from build123d import *

# Parameters (mm, degrees)
F0_R     = 38.89375
F0_R_2   = 6.35
F1_DEPTH = 4.7625
F2_R     = 38.89375
F2_R_2   = 28.575
F3_DEPTH = 1.5875
F4_R     = 6.35
F5_DEPTH = 15.875
F7_DEPTH = 12.7
F7_TAPER = 5
F8_R     = 3.175
F9_DEPTH = 12.7


with BuildPart() as f1:
    # F0 (on Front) → F1 (new body)
    with BuildSketch(Plane.XZ):
        Circle(F0_R)
        Circle(F0_R_2, mode=Mode.SUBTRACT)
    extrude(amount=F1_DEPTH)

    # F2 (on face) → F3 (join)
    with BuildSketch(Plane.XZ.offset(4.7625)):
        Circle(F2_R)
        Circle(F2_R_2, mode=Mode.SUBTRACT)
    extrude(amount=F3_DEPTH)

    # F4 (on face) → F5 (join)
    with BuildSketch(Plane(origin=(0, 0, 0), x_dir=(-1, 0, 0), z_dir=(0, 1, 0))):
        with BuildLine():
            Line((-15.875, -79.375), (15.875, -79.375))
            Line((15.875, -79.375), (15.875, -35.5064524286))
            ThreePointArc((15.875, -35.5064524286), (0, -38.89375), (-15.875, -35.5064524286))
            Line((-15.875, -35.5064524286), (-15.875, -79.375))
        make_face()
        with BuildLine():
            ThreePointArc((-15.875, -35.5064524286), (0, -38.89375), (15.875, -35.5064524286))
            Line((15.875, -35.5064524286), (15.875, 0))
            ThreePointArc((15.875, 0), (4.9e-09, -15.875), (-15.875, -9.8e-09))
            Line((-15.875, -9.8e-09), (-15.875, -35.5064524286))
        make_face()
        with BuildLine():
            ThreePointArc((-15.875, -9.8e-09), (4.9e-09, -15.875), (15.875, 0))
            ThreePointArc((15.875, 0), (-4.9e-09, 15.875), (-15.875, -9.8e-09))
        make_face()
        Circle(F4_R, mode=Mode.SUBTRACT)
    extrude(amount=F5_DEPTH)

    # F6 (on face) → F7 (cut)
    with BuildSketch(Plane(origin=(0, 15.875, 0), x_dir=(-1, 0, 0), z_dir=(0, 1, 0))):
        with BuildLine():
            ThreePointArc((-6.35, -60.325), (-4.4901280605, -64.8151280605), (0, -66.675))
            Line((0, -66.675), (0, -60.325))
            Line((0, -60.325), (-6.35, -60.325))
        make_face()
        with BuildLine():
            Line((0, -60.325), (0, -66.675))
            ThreePointArc((0, -66.675), (4.4901280605, -64.8151280605), (6.35, -60.325))
            Line((6.35, -60.325), (0, -60.325))
        make_face()
        with BuildLine():
            Line((-6.35, -60.325), (0, -60.325))
            Line((0, -60.325), (0, -53.975))
            ThreePointArc((0, -53.975), (-4.4901280605, -55.8348719395), (-6.35, -60.325))
        make_face()
        with BuildLine():
            Line((0, -53.975), (0, -60.325))
            Line((0, -60.325), (6.35, -60.325))
            ThreePointArc((6.35, -60.325), (4.4901280605, -55.8348719395), (0, -53.975))
        make_face()
        with BuildLine():
            Line((-6.35, -22.225), (-6.35, -60.325))
            ThreePointArc((-6.35, -60.325), (-4.4901280605, -55.8348719395), (0, -53.975))
            Line((0, -53.975), (0, -28.575))
            ThreePointArc((0, -28.575), (-4.4901280605, -26.7151280605), (-6.35, -22.225))
        make_face()
        with BuildLine():
            ThreePointArc((0, -53.975), (4.4901280605, -55.8348719395), (6.35, -60.325))
            Line((6.35, -60.325), (6.35, -22.225))
            ThreePointArc((6.35, -22.225), (4.4901280605, -26.7151280605), (0, -28.575))
            Line((0, -28.575), (0, -53.975))
        make_face()
        with BuildLine():
            ThreePointArc((0, -15.875), (-4.4901280605, -17.7348719395), (-6.35, -22.225))
            Line((-6.35, -22.225), (0, -22.225))
            Line((0, -22.225), (0, -15.875))
        make_face()
        with BuildLine():
            Line((0, -22.225), (-6.35, -22.225))
            ThreePointArc((-6.35, -22.225), (-4.4901280605, -26.7151280605), (0, -28.575))
            Line((0, -28.575), (0, -22.225))
        make_face()
        with BuildLine():
            ThreePointArc((0, -28.575), (4.4901280605, -26.7151280605), (6.35, -22.225))
            Line((6.35, -22.225), (0, -22.225))
            Line((0, -22.225), (0, -28.575))
        make_face()
        with BuildLine():
            Line((0, -22.225), (6.35, -22.225))
            ThreePointArc((6.35, -22.225), (4.4901280605, -17.7348719395), (0, -15.875))
            Line((0, -15.875), (0, -22.225))
        make_face()
    extrude(amount=-F7_DEPTH, taper=F7_TAPER, mode=Mode.SUBTRACT)

    # F8 (on face) → F9 (cut)
    with BuildSketch(Plane(origin=(0, 15.875, 0), x_dir=(-1, 0, 0), z_dir=(0, 1, 0))):
        with BuildLine():
            ThreePointArc((3.175, -11.1125), (2.2450640303, -8.8674359697), (0, -7.9375))
            Line((0, -7.9375), (0, -14.2875))
            ThreePointArc((0, -14.2875), (2.2450640303, -13.3575640303), (3.175, -11.1125))
        make_face()
        with BuildLine():
            ThreePointArc((12.7, -69.85), (9.525, -66.675), (6.35, -69.85))
            ThreePointArc((6.35, -69.85), (9.525, -73.025), (12.7, -69.85))
        make_face()
        with Locations((-9.525, -69.85)):
            Circle(F8_R)
        with BuildLine():
            Line((0, -14.2875), (0, -7.9375))
            ThreePointArc((0, -7.9375), (-3.175, -11.1125), (0, -14.2875))
        make_face()
    extrude(amount=-F9_DEPTH, mode=Mode.SUBTRACT)


solid = f1.part
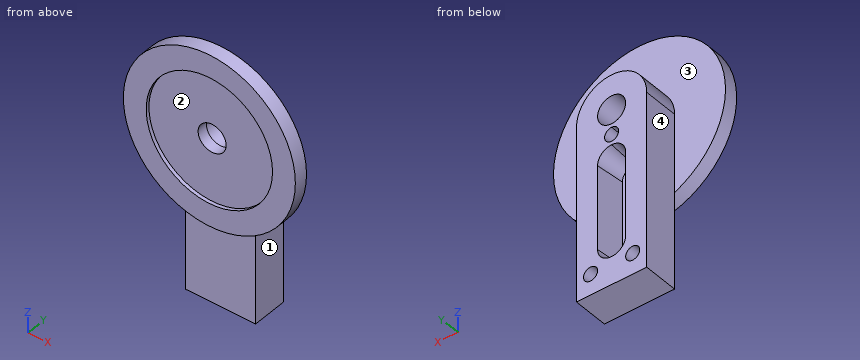
Verification items for the finished model (mm, model axes). Face numbers are marked on the shaded views. Coordinates: 2 decimals unless noted, no trailing zeros. Order: outer loops, then holes, each group sorted by start corner. A loop starts at its lowest first (then second) coordinate and runs counter-clockwise, first axis right, second up. Notation, with made-up numbers: (41, 73.5) -> (82, 73.5) arc R25 cw to (82, 96.5) -> close; hole circle Ø1 at (30, -9). An arc over 180 degrees is marked (long way). Use CSV: the item, a comma, the result in double quotes. Start each with the question number.
Q1. Draft check along X on the marked faces 1, 2, 3 and 4. Enter one of: +X half, -X half, draft (parallel to the pull), parting line (faces both ways), or undercut.
Q2. Section check B-B, the plane z = -69.85. Record the cut outline in (x, y) (3 decimals), and give its area (3 significant figures).
Q3. Thickness scan on line 1 along Z through (x, y) = (0, -5.6) (3 decimals); line 2 along Y through (x, z) = (14, 33); line 3 along Z through (x, y) = (4, 0.75) (3 decimals). Record the ranges inside material, lowest first.
Q4. Section check C-C, the plane y = -2. Record the cut outline in (x, z), and give its area (3 significant figures).
Q5. Depth check by flat-ended pin: P1, Ø4, axis at x = -9.525, z = -69.85, coming from the +Y side (3 decimals); P2, Ø7.5, axis at x = 9.525, z = -69.85, coming from the -Y side; P3, Ø2, axis at y = 3, z = -27.5, coming from the +X side (3 decimals); P4, Ø7.5, axis at x = 0, z = 0, coming from the -Y side. Enter the tip coordinate at first touch or a pass-through.
Q6. Section check D-D, the plane x = 23. Record the cut outline in (y, z), and give its area (3 significant figures).
Returned:
1,face 1,"+X half"
1,face 2,"undercut"
1,face 3,"draft"
1,face 4,"-X half"
2,outline,"(-15.875, 0) -> (15.875, 0) -> (15.875, 15.875) -> (12.7, 15.875) -> (12.7, 3.175) -> (6.35, 3.175) -> (6.35, 15.875) -> (-6.35, 15.875) -> (-6.35, 3.175) -> (-12.7, 3.175) -> (-12.7, 15.875) -> (-15.875, 15.875) -> close"
2,area,"343 mm^2"
3,line 1,"z = -38.894 to -28.575, 28.575 to 38.894"
3,line 2,"y = -6.35 to 0"
3,line 3,"z = -79.375 to -4.932, 4.932 to 15.363"
4,outline,"circle Ø77.79 at (0, 0); hole circle Ø12.7 at (0, 0)"
4,area,"4,630 mm^2"
5,P1,"stops at y = 3.175"
5,P2,"stops at y = 0"
5,P3,"stops at x = 15.875"
5,P4,"passes through"
6,outline,"(-6.35, -31.36) -> (0, -31.36) -> (0, 31.36) -> (-6.35, 31.36) -> (-6.35, 16.96) -> (-4.76, 16.96) -> (-4.76, -16.96) -> (-6.35, -16.96) -> close"
6,area,"344 mm^2"
